Autodesk Inventor part; units mm, degrees
ref_plane "YZ Plane" through (0, 0, 0) normal (1, 0, 0) x (0, 1, 0)
ref_plane "XZ Plane" through (0, 0, 0) normal (0, 1, 0) x (-1, 0, 0)
ref_plane "XY Plane" through (0, 0, 0) normal (0, 0, 1) x (1, 0, 0)
sketch "Szkic1" plane through (0, 0, 0) normal (0, 1, 0) x (-1, 0, 0)
  line L0 (-20, -8) -> (20, -8)
  line L1 (20, -8) -> (20, 8)
  line L2 (20, 8) -> (-20, 8)
  line L3 (-20, 8) -> (-20, -8)
  line L4 (-20, -8) -> (20, 8) construction
  line L5 (20, -8) -> (-20, 8) construction
  point P0 (0, 0)
  dimension "d0" = 40
  dimension "d1" = 16
extrude "Wyciągnięcie proste1" add sketch "Szkic1" along normal blind 1
sketch "Szkic2" plane through (0, 0, 0) normal (0, -1, 0) x (1, 0, 0)
  circle A0 centre (-12, 0) radius 6
  circle A1 centre (12, 0) radius 6
  point P0 (0, 0)
  dimension "d4" = 12
  dimension "d5" = 12
extrude "Wyciągnięcie proste2" add sketch "Szkic2" along normal blind 10
sketch "Szkic3" plane through (0, 0, 0) normal (0, -1, 0) x (1, 0, 0)
  line L0 (20, -8) -> (-20, -8)
  line L1 (2, -5.5) -> (-2, -5.5) construction
  line L2 (2, -4.5) -> (-2, -4.5)
  line L3 (-2, -6.5) -> (2, -6.5)
  arc A0 (2, -6.5) -> (2, -4.5) centre (2, -5.5) ccw
  arc A1 (-2, -4.5) -> (-2, -6.5) centre (-2, -5.5) ccw
  point P0 (0, 0)
  point P1 (0, -5.5)
  dimension "d8" = 4
  dimension "d9" = 2
extrude "Wyciągnięcie proste3" add sketch "Szkic3" along normal blind 2
chamfer "Faza1" distance 0.5 angle 45 1 edges at (-18, -10, 0)
chamfer "Faza2" distance 0.5 angle 45 1 edges at (6, -10, 0)
chamfer "Faza3" distance 0.2 angle 45 4 edges at (0, -2, -6.5) (3, -2, -5.5) (0, -2, -4.5) (-3, -2, -5.5)
chamfer "Faza4" distance 0.2 angle 45 1 edges at (0, 0, 8)
chamfer "Faza5" distance 0.2 angle 45 1 edges at (-20, 0, -0.1)
chamfer "Faza6" distance 0.2 angle 45 1 edges at (0.1, 0, -8)
chamfer "Faza7" distance 0.2 angle 45 1 edges at (20, 0, 0)
chamfer "Faza8" distance 0.2 angle 45 1 edges at (0, 1, 8)
chamfer "Faza9" distance 0.2 angle 45 1 edges at (20, 1, -0.1)
chamfer "Faza10" distance 0.2 angle 45 1 edges at (-0.1, 1, -8)
chamfer "Faza11" distance 0.2 angle 45 1 edges at (-20, 1, 0)
sketch "Szkic4" plane through (0, 1, 0) normal (0, 1, 0) x (1, 0, 0)
  line L0 (-17.7792, 4.1723) -> (-14.2918, 4.1723)
  line L1 (-14.2918, 4.1723) -> (-14.2918, -3.3005)
  line L2 (-14.2918, -3.3005) -> (-17.7792, -3.3005)
  line L3 (-17.7792, -3.3005) -> (-17.7792, 4.1723)
  line L4 (-17.7792, 4.1723) -> (-14.2918, -3.3005) construction
  line L5 (-14.2918, 4.1723) -> (-17.7792, -3.3005) construction
  line L6 (-9.9327, 3.7987) -> (-1.9616, 3.7987)
  line L7 (-1.9616, 3.7987) -> (-1.9616, -0.4359)
  line L8 (-1.9616, -0.4359) -> (-9.9327, -0.4359)
  line L9 (-9.9327, -0.4359) -> (-9.9327, 3.7987)
  line L10 (-9.9327, 3.7987) -> (-1.9616, -0.4359) construction
  line L11 (-1.9616, 3.7987) -> (-9.9327, -0.4359) construction
  line L12 (10.3063, -4.1101) -> (5.8226, -4.1101)
  line L13 (5.8226, -4.1101) -> (5.8226, 3.2382)
  line L14 (5.8226, 3.2382) -> (10.3063, 3.2382)
  line L15 (10.3063, 3.2382) -> (10.3063, -4.1101)
  line L16 (10.3063, -4.1101) -> (5.8226, 3.2382) construction
  line L17 (5.8226, -4.1101) -> (10.3063, 3.2382) construction
  point P0 (0, 0)
  point P1 (-16.0355, 0.4359)
  point P2 (-5.9471, 1.6814)
  point P3 (8.0645, -0.4359)
extrude "Wyciągnięcie proste4" add sketch "Szkic4" along normal blind 1
chamfer "Faza12" distance 0.2 angle 45 13 edges at (-5.9471, 2, 0.4359) (-1.9616, 2, -1.6814) (-5.9471, 2, -3.7987) (-9.9327, 2, -1.6814) (-14.2918, 2, -0.4359) (-16.0355, 2, 3.3005) (-17.7792, 2, -0.4359) (-16.0355, 2, -4.1723) (8.0645, 2, 4.1101) (5.8226, 1, 0.4359) (10.3063, 2, 0.4359) (8.0645, 2, -3.2382) (5.8226, 2, 0.4359)
sketch "Szkic5" plane through (-12, -10, 0) normal (0, -1, 0) x (1, 0, 0)
  circle A0 centre (0, 0) radius 5.5
  circle A1 centre (24, 0) radius 5.5
  point P0 (12, 0)
sketch "Szkic6" plane through (-12, -10, 0) normal (0, -1, 0) x (1, 0, 0)
  circle A0 centre (0, 0) radius 5.5
  circle A1 centre (0, 0) radius 4.5
  point P0 (12, 0)
  dimension "d50" = 9
extrude "Wyciągnięcie proste5" cut sketch "Szkic6" against normal blind 7 contours A1
chamfer "Faza13" distance 0.5 angle 45 1 edges at (-16.5, -10, 0)
sketch "Szkic7" plane through (12, -10, 0) normal (0, -1, 0) x (1, 0, 0)
  circle A0 centre (0, 0) radius 5.5
  circle A1 centre (0, 0) radius 4.5
  point P0 (-12, 0)
  dimension "d56" = 9
extrude "Wyciągnięcie proste6" cut sketch "Szkic7" against normal blind 7 contours A1
chamfer "Faza14" distance 0.5 angle 45 1 edges at (7.5, -10, 0)
sketch "Szkic8" plane through (0, 1, 0) normal (0, 1, 0) x (1, 0, 0)
  line L0 (-2.5, -7.625) -> (2.5, -7.625)
  line L1 (2.5, -7.625) -> (2.5, -6.375)
  line L2 (2.5, -6.375) -> (-2.5, -6.375)
  line L3 (-2.5, -6.375) -> (-2.5, -7.625)
  line L4 (-2.5, -7.625) -> (2.5, -6.375) construction
  line L5 (2.5, -7.625) -> (-2.5, -6.375) construction
  point P0 (0, 0)
  point P1 (0, -7)
  dimension "d62" = 5
  dimension "d63" = 1.25
extrude "Wyciągnięcie proste7" add sketch "Szkic8" along normal blind 1
sketch "Szkic9" plane through (-2.5, 1, 7.625) normal (0, 0, 1) x (1, 0, 0)
  line L0 (0.9, 0.7) -> (0.5, 0.7)
  line L1 (0.5, 0.7) -> (0.5, 0.3)
  line L2 (0.5, 0.3) -> (0.9, 0.3)
  line L3 (0.9, 0.3) -> (0.9, 0.7)
  line L4 (0.9, 0.7) -> (0.5, 0.3) construction
  line L5 (0.5, 0.7) -> (0.9, 0.3) construction
  line L6 (4.1, 0.7) -> (4.5, 0.7)
  line L7 (4.5, 0.7) -> (4.5, 0.3)
  line L8 (4.5, 0.3) -> (4.1, 0.3)
  line L9 (4.1, 0.3) -> (4.1, 0.7)
  line L10 (4.1, 0.7) -> (4.5, 0.3) construction
  line L11 (4.5, 0.7) -> (4.1, 0.3) construction
  line L12 (2.1, 0.7) -> (1.7, 0.7)
  line L13 (1.7, 0.7) -> (1.7, 0.3)
  line L14 (1.7, 0.3) -> (2.1, 0.3)
  line L15 (2.1, 0.3) -> (2.1, 0.7)
  line L16 (2.1, 0.7) -> (1.7, 0.3) construction
  line L17 (1.7, 0.7) -> (2.1, 0.3) construction
  line L18 (2.9, 0.7) -> (3.3, 0.7)
  line L19 (3.3, 0.7) -> (3.3, 0.3)
  line L20 (3.3, 0.3) -> (2.9, 0.3)
  line L21 (2.9, 0.3) -> (2.9, 0.7)
  line L22 (2.9, 0.7) -> (3.3, 0.3) construction
  line L23 (3.3, 0.7) -> (2.9, 0.3) construction
  point P0 (2.5, -1)
  point P1 (0.7, 0.5)
  point P2 (4.3, 0.5)
  point P3 (1.9, 0.5)
  point P4 (3.1, 0.5)
  dimension "d66" = 0.4
  dimension "d67" = 0.4
  dimension "d68" = 0.4
  dimension "d69" = 0.4
  dimension "d70" = 0.4
  dimension "d71" = 0.4
  dimension "d72" = 0.4
  dimension "d73" = 0.4
extrude "Wyciągnięcie proste8" add sketch "Szkic9" along normal blind 6
chamfer "Faza15" distance 0.15 angle 45 4 edges at (-2, 1.5, 13.625) (-1.8, 1.3, 13.625) (-1.6, 1.5, 13.625) (-1.8, 1.7, 13.625)
chamfer "Faza16" distance 0.15 angle 45 12 edges at (-0.6, 1.7, 13.625) (-0.8, 1.5, 13.625) (-0.6, 1.3, 13.625) (-0.4, 1.5, 13.625) (0.6, 1.3, 13.625) (0.8, 1.5, 13.625) (0.6, 1.7, 13.625) (0.4, 1.5, 13.625) (1.6, 1.5, 13.625) (1.8, 1.3, 13.625) (2, 1.5, 13.625) (1.8, 1.7, 13.625)
properties part number "czujnik_ultra_dzwiek" material "Kauczuk, silikon"
Could you check a few things on this model? Use its own coordinates, in mm. A direction names the side the tool comes from. Coordinates: 2 decimals unless noted, no trailing zeros. Order: outer loops, then holes, each group sorted by start corner. A loop starts at its lowest first (then second) coordinate and runs counter-clockwise, first axis right, second up. Notation, with made-up numbers: M 4,46.25 L 24,46.25 A22 ccw 24,62.25 Z; hole C -14,14 d7. An arc over 180 degrees is marked long. Use one line per item in the form item = value. Start each with the question number.
1. For pin 1 (4.5 mm diameter, centred on x = -14, z = -0.5, fed in from -Y); pin 2 (6 mm diameter, centred on y = -7.5, z = -3, fed in from -X); pin 3 (2 mm diameter, centred on x = -8, z = 7, fed in from -Y), each with a flat end and sliding along its axis, tell me the tip position at first contact or that it passes through.
2. Suppose I cut it at C-C on x = -12. Write out the boundary of the cut face in (y, z), then the cut area to 3 significant figures.
3. Suppose I cut it at D-D on z = 7. Write out the boundary of the cut face in (x, y), then the cut area to 3 significant figures.
4. Suppose I cut it at B-B on y = -7.75. Write out the boundary of the cut face in (x, z).
5. Suppose I cut it at A-A on z = 9.25. Write out the boundary of the cut face in (x, y), then the cut area to 3 significant figures.
6. We'd pull the mould along X, two halves only. Please class faces 1 (the flat face through (0, -1, -4.5)), 2 (the flat face through (2.5, 1.5, 7)), 3 (the cylindrical face through (3, -0.9, -5.5)), 4 (the flat face through (-10.4, -10, -4.9)): +X half, -X half, draft (parallel to the pull), parting line (faces both ways), or undercut.
7. On a 3-axis mill with a long thin cutter (end or side, diameter ignored), from which of +Z, -Z, +X, -X, +Y, -Y can I reach the whole of each face in a straight line? I mean faces 5 (the cylindrical face through (-7.708, -6.296, 1.352)), 6 (the flat face through (0, 2, 7)), 7 (the flat face through (13.6, -10, -4.9)), 8 (the flat face through (0, -1, -6.5)), 9 (the flat face through (-2.5, 1.5, 7)). Say none if no direction works.
8. Please list where these lines run through material, in increasing order: line 1 (Z direction, x = -12, y = -4.75); line 2 (X direction, y = -7, z = -3); line 3 (X direction, y = -6, z = 1.5).
Geometry says:
q1.pin_1 = -3
q1.pin_2 = -18
q1.pin_3 = 0
q2.outline = M -10,-5.5 L -9.5,-6 L 0,-6 L 0,-7.8 L 0.2,-8 L 0.8,-8 L 1,-7.8 L 1,7.8 L 0.8,8 L 0.2,8 L 0,7.8 L 0,6 L -9.5,6 L -10,5.5 L -10,5 L -9.5,4.5 L -3,4.5 L -3,-4.5 L -9.5,-4.5 L -10,-5 Z
q2.area = 72.4 mm^2
q3.outline = M -20,0.2 L -19.8,0 L 19.8,0 L 20,0.2 L 20,0.8 L 19.8,1 L 2.5,1 L 2.5,2 L -2.5,2 L -2.5,1 L -19.8,1 L -20,0.8 Z
q3.area = 44.9 mm^2
q4.outline = C -12,0 d12; C 12,0 d12; hole C -12,0 d9; hole C 12,0 d9
q5.outline = M -2,1.3 L -1.6,1.3 L -1.6,1.7 L -2,1.7 Z; M -0.8,1.3 L -0.4,1.3 L -0.4,1.7 L -0.8,1.7 Z; M 0.4,1.3 L 0.8,1.3 L 0.8,1.7 L 0.4,1.7 Z; M 1.6,1.3 L 2,1.3 L 2,1.7 L 1.6,1.7 Z
q5.area = 0.640 mm^2
q6.face_1 = undercut
q6.face_2 = +X half
q6.face_3 = undercut
q6.face_4 = draft
q7.face_5 = -Y
q7.face_6 = +Z, -Z, +X, -X, +Y
q7.face_7 = +Z, -Z, +X, -X, -Y
q7.face_8 = -Z, +X, -X, -Y
q7.face_9 = +Z, -X, +Y
q8.line_1 = -6 to -4.5, 4.5 to 6
q8.line_2 = -17.2 to -15.35, -8.65 to -6.8, 6.8 to 8.65, 15.35 to 17.2
q8.line_3 = -17.81 to -16.24, -7.76 to -6.19, 6.19 to 7.76, 16.24 to 17.81
